from build123d import *

# Parameters (mm, degrees)
SKETCH1_W           = 25.4
SKETCH1_H           = 25.4
BOSS_EXTRUDE1_DEPTH = 1
SKETCH2_W           = 22.8
SKETCH2_H           = 22.8
SKETCH2_W_2         = 18.8
SKETCH2_H_2         = 18.8
BOSS_EXTRUDE2_DEPTH = 4
FILLET1_R           = 2
SKETCH3_W           = 1.3
SKETCH3_H           = 3.6
CUT_EXTRUDE1_DEPTH  = 19.643497526
BOSS_EXTRUDE3_START = 4
BOSS_EXTRUDE3_DEPTH = 4


with BuildPart() as part:
    # Sketch1 → Boss-Extrude1 (new body)
    with BuildSketch(Plane(origin=(0, 0, 0), x_dir=(1, 0, 0), z_dir=(0, 1, 0))):
        Rectangle(SKETCH1_W, SKETCH1_H)
    extrude(amount=BOSS_EXTRUDE1_DEPTH)

    # Sketch2 → Boss-Extrude2 (add)
    with BuildSketch(Plane(origin=(0, 1, 0), x_dir=(1, 0, 0), z_dir=(0, 1, 0))):
        Rectangle(SKETCH2_W, SKETCH2_H)
        Rectangle(SKETCH2_W_2, SKETCH2_H_2, mode=Mode.SUBTRACT)
    extrude(amount=BOSS_EXTRUDE2_DEPTH)

    # Fillet1
    fillet1_edges = [part.edges().sort_by_distance(p)[0] for p in [
        (11.4, 3, 11.4),
        (11.4, 3, -11.4),
        (-11.4, 3, -11.4),
        (-11.4, 3, 11.4),
        (-9.4, 3, -9.4),
        (-9.4, 3, 9.4),
        (9.4, 3, 9.4),
        (9.4, 3, -9.4),
    ]]
    fillet(fillet1_edges, radius=FILLET1_R)

    # Sketch3 → Cut-Extrude1 (cut, through all)
    with BuildSketch(Plane(origin=(0, 5, 0), x_dir=(1, 0, 0), z_dir=(0, 1, 0))):
        with BuildLine():
            Line((-6.7, 1.8), (-9.1, 1.8))
            ThreePointArc((-9.1, 1.8), (-9.261854267, 1.561058204), (-9.4, 1.307669683))
            Line((-9.4, 1.307669683), (-9.4, -1.307669683))
            ThreePointArc((-9.4, -1.307669683), (-9.261854267, -1.561058204), (-9.1, -1.8))
            Line((-9.1, -1.8), (-6.7, -1.8))
            Line((-6.7, -1.8), (-6.7, 1.8))
        make_face()
        with Locations((-12.05, 0)):
            Rectangle(SKETCH3_W, SKETCH3_H)
        with BuildLine():
            Line((-9.4, 1.8), (-11.4, 1.8))
            Line((-11.4, 1.8), (-11.4, -1.8))
            Line((-11.4, -1.8), (-9.4, -1.8))
            Line((-9.4, -1.8), (-9.4, -1.307669683))
            ThreePointArc((-9.4, -1.307669683), (-9.7, 0), (-9.4, 1.307669683))
            Line((-9.4, 1.307669683), (-9.4, 1.8))
        make_face()
        with BuildLine():
            ThreePointArc((-3.7, 0), (-5.751316702, 2.846049894), (-9.1, 1.8))
            Line((-9.1, 1.8), (-6.7, 1.8))
            Line((-6.7, 1.8), (-6.7, -1.8))
            Line((-6.7, -1.8), (-9.1, -1.8))
            ThreePointArc((-9.1, -1.8), (-5.751316702, -2.846049894), (-3.7, 0))
        make_face()
        with BuildLine():
            Line((-9.1, 1.8), (-9.4, 1.8))
            Line((-9.4, 1.8), (-9.4, 1.307669683))
            ThreePointArc((-9.4, 1.307669683), (-9.261854267, 1.561058204), (-9.1, 1.8))
        make_face()
        with BuildLine():
            Line((-9.4, -1.307669683), (-9.4, 1.307669683))
            ThreePointArc((-9.4, 1.307669683), (-9.7, 0), (-9.4, -1.307669683))
        make_face()
        with BuildLine():
            Line((-9.4, -1.307669683), (-9.4, -1.8))
            Line((-9.4, -1.8), (-9.1, -1.8))
            ThreePointArc((-9.1, -1.8), (-9.261854267, -1.561058204), (-9.4, -1.307669683))
        make_face()
    extrude(amount=-CUT_EXTRUDE1_DEPTH, mode=Mode.SUBTRACT)

    # Sketch4 → Boss-Extrude3 (add)
    with BuildSketch(Plane(origin=(0, 1, 0), x_dir=(1, 0, 0), z_dir=(0, 1, 0)).offset(BOSS_EXTRUDE3_START)):
        with BuildLine():
            Line((-9.1, 1.8), (-9.4, 1.8))
            Line((-9.4, 1.8), (-9.4, 2.951270913))
            ThreePointArc((-9.4, 2.951270913), (-2.7, 0), (-9.4, -2.951270913))
            Line((-9.4, -2.951270913), (-9.4, -1.8))
            Line((-9.4, -1.8), (-9.1, -1.8))
            ThreePointArc((-9.1, -1.8), (-3.7, 0), (-9.1, 1.8))
        make_face()
    extrude(amount=-BOSS_EXTRUDE3_DEPTH)


solid = part.part
Geometry: final body of the model. Coordinates: model frame, mm. A direction names the side the tool comes from. Give positions to 0.01 mm unless a question says otherwise; leave off trailing zeros. Order: outer loops, then holes, each group sorted by start corner. A loop starts at its lowest first (then second) coordinate and runs counter-clockwise, first axis right, second up. Notation, with made-up numbers: (71, -19) - (101, -19) arc R26 ccw to (101, 16) - close; hole circle Ø6 at (36.5, 61). An arc over 180 degrees is marked (long way). Use CSV: the item, a comma, the result in double quotes.
1. Material intervals for line 1 along Z through (x, y) = (-6.7, 2.4); line 2 along X through (y, z) = (2.8, 5.25); line 3 along X through (y, z) = (1.8, 0), sorted ascending. Write a range as from..to.
Answers below:
line 1,"-11.4..-9.4, -4..-3, 3..4, 9.4..11.4"
line 2,"-11.4..-9.4, 9.4..11.4"
line 3,"-3.7..-2.7, 9.4..11.4"
2. Section query A-A (y = 3.1). Output: boundary loops of the cut face in (x, z), plus the area to 3 significant figures.
Answers below:
outline,"(-11.4, -9.4) arc R2 ccw to (-9.4, -11.4) - (9.4, -11.4) arc R2 ccw to (11.4, -9.4) - (11.4, 9.4) arc R2 ccw to (9.4, 11.4) - (-9.4, 11.4) arc R2 ccw to (-11.4, 9.4) - (-11.4, 1.8) - (-9.1, 1.8) arc R3 cw (long way) to (-9.1, -1.8) - (-11.4, -1.8) - close; hole (-9.4, -7.4) arc R2 ccw to (-7.4, -9.4) - (7.4, -9.4) arc R2 ccw to (9.4, -7.4) - (9.4, 7.4) arc R2 ccw to (7.4, 9.4) - (-7.4, 9.4) arc R2 ccw to (-9.4, 7.4) - (-9.4, 2.95) arc R4 cw (long way) to (-9.4, -2.95) - close"
area,"176 mm2"
3. Section query B-B (x = -6.7). Output: boundary loops of the cut face in (y, z), plus the area to 3 significant figures.
Answers below:
outline,"(0, -12.7) - (1, -12.7) - (1, -11.4) - (5, -11.4) - (5, -9.4) - (1, -9.4) - (1, -4) - (5, -4) - (5, -3) - (0, -3) - close; (0, 3) - (5, 3) - (5, 4) - (1, 4) - (1, 9.4) - (5, 9.4) - (5, 11.4) - (1, 11.4) - (1, 12.7) - (0, 12.7) - close"
area,"43.4 mm2"
4. Section query D-D (z = 5). Output: boundary loops of the cut face in (x, y).
Answers below:
outline,"(-12.7, 0) - (12.7, 0) - (12.7, 1) - (11.4, 1) - (11.4, 5) - (9.4, 5) - (9.4, 1) - (-9.4, 1) - (-9.4, 5) - (-11.4, 5) - (-11.4, 1) - (-12.7, 1) - close"
5. Section query C-C (z = 2.25). Output: boundary loops of the cut face in (x, y), plus the area to 3 significant figures.
Answers below:
outline,"(-12.7, 0) - (-8.68, 0) - (-8.68, 5) - (-11.4, 5) - (-11.4, 1) - (-12.7, 1) - close; (-4.72, 0) - (12.7, 0) - (12.7, 1) - (11.4, 1) - (11.4, 5) - (9.4, 5) - (9.4, 1) - (-3.39, 1) - (-3.39, 5) - (-4.72, 5) - close"
area,"45.6 mm2"
6. Contact query for flat-ended pins moving along their axis: pin 1 (1.5 mm diameter, centred on x = -6, y = 2, fed in from +Z); pin 2 (3 mm diameter, centred on x = 5, y = 3, fed in from -Z); pin 3 (2 mm diameter, centred on y = 4, z = -4.5, fed in from +X); pin 4 (1.5 mm diameter, centred on x = -9, z = 1, fed in from -Y). Output: stop coordinate, or through.
Answers below:
pin 1,"z = 11.4"
pin 2,"z = -11.4"
pin 3,"x = 11.4"
pin 4,"through"
7. Access query for faces 4 (the face through (10.83, 3.03, -10.8)), 5 (the face through (-10.8, 3.03, -10.83)), 6 (the face through (8.8, 3.03, 8.83)), 7 (the face through (11.4, 3, 0)). Directions: +Z, -Z, +X, -X, +Y, -Y. A direction counts if a zero-diameter tool reaches every point of the face in a straight line with its end or side. Return the directions, or none.
Answers below:
face 4,"-Z, +X, +Y"
face 5,"-Z, -X, +Y"
face 6,"+Y"
face 7,"+Z, -Z, +X, +Y"
8. Mould query, pull axis X, two halves, no side actions, for faces 1 (the face through (0, 0, 0)), 2 (the face through (-9.4, 3, 5)), 3 (the face through (-11.4, 3, 6)). Classes: +X half, -X half, draft (parallel to the pull), parting line (faces both ways), or undercut.
Answers below:
face 1,"draft"
face 2,"undercut"
face 3,"-X half"
